The listing builds one solid part. Answer for the finished solid, in the listing's coordinates (mm). Face numbers are marked on the shaded views. A direction names the side the tool comes from. Coordinates: 2 decimals unless noted, no trailing zeros. Order: outer loops, then holes, each group sorted by start corner. A loop starts at its lowest first (then second) coordinate and runs counter-clockwise, first axis right, second up. Notation, with made-up numbers: (71, 17) -> (75, 17) arc R15 ccw to (75, 35) -> close; hole circle Ø4 at (63, 27.5). An arc over 180 degrees is marked (long way). Return JSON: item names as keys, results as strings.
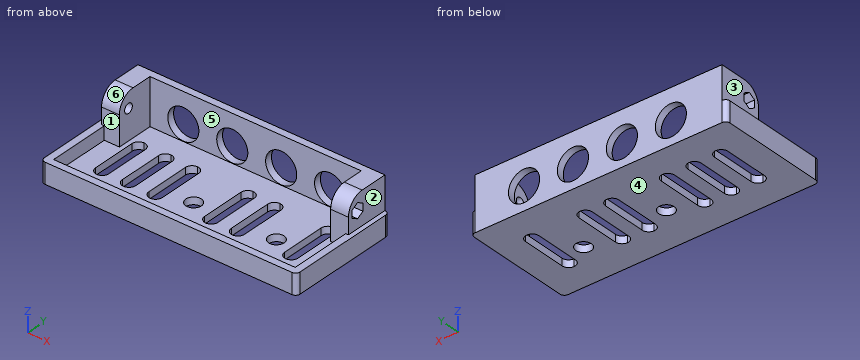
```python
from build123d import *

# Parameters (mm, degrees)
F0_W      = 115
F0_H      = 51
F0_R      = 3.5
F1_DEPTH  = 3.2
F3_DEPTH  = 24
F5_DEPTH  = 6
F6_R      = 2.125
F7_DEPTH  = 113.001
F8_R      = 7.5
F9_R      = 2
F10_R     = 7
F11_DEPTH = 5
F13_DEPTH = 4


# Not quite as in the source:
# - a pattern or mirror of a feature is missing from the dataset's text; its kind, count and spacing are read off the source's solid


with BuildPart() as f1:
    # F0 (on Top) → F1 (new body)
    with BuildSketch(Plane.XY):
        Rectangle(F0_W, F0_H)
        with BuildLine():
            Line((-39.5, 10), (-39.5, -10))
            ThreePointArc((-39.5, -10), (-40.3786796564, -12.1213203436), (-42.5, -13))
            ThreePointArc((-42.5, -13), (-44.6213203436, -12.1213203436), (-45.5, -10))
            Line((-45.5, -10), (-45.5, 10))
            ThreePointArc((-45.5, 10), (-44.6213203436, 12.1213203436), (-42.5, 13))
            ThreePointArc((-42.5, 13), (-40.3786796564, 12.1213203436), (-39.5, 10))
        make_face(mode=Mode.SUBTRACT)
        with Locations((-5.112, -5.5)):
            Circle(F0_R, mode=Mode.SUBTRACT)
        with Locations((32.1, -5.5)):
            Circle(F0_R, mode=Mode.SUBTRACT)
        with BuildLine():
            Line((-27.5, 10), (-27.5, -10))
            ThreePointArc((-27.5, -10), (-28.3786796564, -12.1213203436), (-30.5, -13))
            ThreePointArc((-30.5, -13), (-32.6213203436, -12.1213203436), (-33.5, -10))
            Line((-33.5, -10), (-33.5, 10))
            ThreePointArc((-33.5, 10), (-32.6213203436, 12.1213203436), (-30.5, 13))
            ThreePointArc((-30.5, 13), (-28.3786796564, 12.1213203436), (-27.5, 10))
        make_face(mode=Mode.SUBTRACT)
        with BuildLine():
            Line((-15.5, 10), (-15.5, -10))
            ThreePointArc((-15.5, -10), (-16.3786796564, -12.1213203436), (-18.5, -13))
            ThreePointArc((-18.5, -13), (-20.6213203436, -12.1213203436), (-21.5, -10))
            Line((-21.5, -10), (-21.5, 10))
            ThreePointArc((-21.5, 10), (-20.6213203436, 12.1213203436), (-18.5, 13))
            ThreePointArc((-18.5, 13), (-16.3786796564, 12.1213203436), (-15.5, 10))
        make_face(mode=Mode.SUBTRACT)
        with BuildLine():
            Line((9.5, 10), (9.5, -10))
            ThreePointArc((9.5, -10), (8.6213203436, -12.1213203436), (6.5, -13))
            ThreePointArc((6.5, -13), (4.3786796564, -12.1213203436), (3.5, -10))
            Line((3.5, -10), (3.5, 10))
            ThreePointArc((3.5, 10), (4.3786796564, 12.1213203436), (6.5, 13))
            ThreePointArc((6.5, 13), (8.6213203436, 12.1213203436), (9.5, 10))
        make_face(mode=Mode.SUBTRACT)
        with BuildLine():
            Line((21.5, 10), (21.5, -10))
            ThreePointArc((21.5, -10), (20.6213203436, -12.1213203436), (18.5, -13))
            ThreePointArc((18.5, -13), (16.3786796564, -12.1213203436), (15.5, -10))
            Line((15.5, -10), (15.5, 10))
            ThreePointArc((15.5, 10), (16.3786796564, 12.1213203436), (18.5, 13))
            ThreePointArc((18.5, 13), (20.6213203436, 12.1213203436), (21.5, 10))
        make_face(mode=Mode.SUBTRACT)
        with BuildLine():
            Line((45.5, 10), (45.5, -10))
            ThreePointArc((45.5, -10), (44.6213203436, -12.1213203436), (42.5, -13))
            ThreePointArc((42.5, -13), (40.3786796564, -12.1213203436), (39.5, -10))
            Line((39.5, -10), (39.5, 10))
            ThreePointArc((39.5, 10), (40.3786796564, 12.1213203436), (42.5, 13))
            ThreePointArc((42.5, 13), (44.6213203436, 12.1213203436), (45.5, 10))
        make_face(mode=Mode.SUBTRACT)
    extrude(amount=F1_DEPTH)

    # F2 (on face) → F3 (join)
    with BuildSketch(Plane(origin=(0, 0, 0), x_dir=(1, 0, 0), z_dir=(0, 0, -1))):
        Polygon((-47.5, -5.5), (-55.5, -5.5), (-55.5, -25.5), (55.5, -25.5), (55.5, -5.5), (47.5, -5.5), (47.5, -22.3), (-47.5, -22.3), align=None)
    extrude(amount=-F3_DEPTH)

    # F4 (on face) → F5 (join)
    with BuildSketch(Plane.XY.offset(3.2)):
        Polygon((-55.5, 5.5), (-55.5, 25.5), (-57.5, 25.5), (-57.5, -25.5), (57.5, -25.5), (57.5, 25.5), (55.5, 25.5), (55.5, 5.5), (54.3, 5.5), (54.3, -22.3), (-54.3, -22.3), (-54.3, 5.5), align=None)
    extrude(amount=F5_DEPTH)

    # F6 (on face) → F7 (cut, through all)
    with BuildSketch(Plane.YZ.offset(55.5)):
        with Locations((10.5, 16.7)):
            Circle(F6_R)
    extrude(amount=-F7_DEPTH, mode=Mode.SUBTRACT)

    # F8
    f8_edges = [f1.edges().sort_by_distance(p)[0] for p in [
        (51.5, 5.5, 24),
        (-51.5, 5.5, 24),
    ]]
    fillet(f8_edges, radius=F8_R)

    # F9
    f9_edges = [f1.edges().sort_by_distance(p)[0] for p in [
        (-57.5, -25.5, 4.6),
        (57.5, -25.5, 4.6),
        (57.5, 25.5, 4.6),
        (-57.5, 25.5, 4.6),
    ]]
    fillet(f9_edges, radius=F9_R)

    # F10 (on face) → F11 (cut)
    with BuildSketch(Plane(origin=(0, 25.5, 0), x_dir=(-1, 0, 0), z_dir=(0, 1, 0))):
        with Locations((-33.5, 10.4)):
            Circle(F10_R)
        with Locations((-11.5, 10.4)):
            Circle(F10_R)
        with Locations((10.5, 10.4)):
            Circle(F10_R)
        with Locations((32.5, 10.4)):
            Circle(F10_R)
    extrude(amount=-F11_DEPTH, mode=Mode.SUBTRACT)

    # F12 (on face) → F13 (cut)
    with BuildSketch(Plane(origin=(-55.5, 0, 0), x_dir=(0, -1, 0), z_dir=(-1, 0, 0))):
        Polygon((-7.575, 15.0112504626), (-7.575, 18.3887495374), (-10.5, 20.0774990748), (-13.425, 18.3887495374), (-13.425, 15.0112504626), (-10.5, 13.3225009252), align=None)
    f13 = extrude(amount=-F13_DEPTH, mode=Mode.SUBTRACT)

    # F13_copies: F13 across plane
    add(f13.mirror(Plane(origin=(0, 0, 0), x_dir=(0, 0, 1), z_dir=(1, 0, 0))), mode=Mode.SUBTRACT)


solid = f1.part
```
Item 1: The part is cut by section B-B on y = 0. Count the separate pieces of the cut face and the enclosed holes in it, plus the area to 3 significant figures.
Answer list:
{"separate pieces": "7", "enclosed holes": "0", "area": "291 mm2"}
Item 2: The part is cut by section C-C on x = 33.5. Determine the outline of the cut face in (y, z), plus the area to 3 significant figures.
Answer list:
{"outline": "(-25.5, 0) -> (-8.71, 0) -> (-8.71, 3.2) -> (-22.3, 3.2) -> (-22.3, 9.2) -> (-25.5, 9.2) -> close; (-2.29, 0) -> (25.5, 0) -> (25.5, 3.4) -> (22.3, 3.4) -> (22.3, 3.2) -> (-2.29, 3.2) -> close; (22.3, 17.4) -> (25.5, 17.4) -> (25.5, 24) -> (22.3, 24) -> close", "area": "184 mm2"}
Item 3: Find the intervals of material crossed by probe 1 along Y at (x, z) = (6, 4); probe 2 along X at (y, z) = (8.5, 8.25); probe 3 along X at (y, z) = (18, 14.5), in increasing order.
Answer list:
{"probe 1": "-25.5 to -22.3, 22.3 to 25.5", "probe 2": "-57.5 to -47.5, 47.5 to 57.5", "probe 3": "-55.5 to -47.5, 47.5 to 55.5"}
Item 4: Flat-ended cylindrical pins translate along their axes: pin 1 (6 mm diameter, centred on x = 22.5, y = 13.5, fed in from +Z); pin 2 (8.5 mm diameter, centred on x = -10.5, z = 10.4, fed in from +Y); pin 3 (3 mm diameter, centred on x = 12, z = 21.5, fed in from -Y); pin 4 (6 mm diameter, centred on y = -2.5, z = 14, fed in from +X). Find the tip coordinate at first contact, or state that the pin passes through.
Answer list:
{"pin 1": "z = 3.2", "pin 2": "y = -22.3", "pin 3": "y = 22.3", "pin 4": "through"}
Item 5: The part is cut by section A-A on x = 11.5. Determine the outline of the cut face in (y, z).
Answer list:
{"outline": "(-25.5, 0) -> (25.5, 0) -> (25.5, 3.4) -> (22.3, 3.4) -> (22.3, 3.2) -> (-22.3, 3.2) -> (-22.3, 9.2) -> (-25.5, 9.2) -> close; (22.3, 17.4) -> (25.5, 17.4) -> (25.5, 24) -> (22.3, 24) -> close"}
Item 6: The part is cut by section D-D on y = -20. Determine the outline of the cut face in (x, z).
Answer list:
{"outline": "(-57.5, 0) -> (57.5, 0) -> (57.5, 9.2) -> (54.3, 9.2) -> (54.3, 3.2) -> (-54.3, 3.2) -> (-54.3, 9.2) -> (-57.5, 9.2) -> close"}
Item 7: Which of the six approach directions +Z, -Z, +X, -X, +Y, -Y give full straight-line access (tool end or side, diameter ignored) to the marked faces 1, 2 and 3?
Answer list:
{"face 1": "+Z", "face 2": "+Z, +X, +Y, -Y", "face 3": "+Z, -X, +Y, -Y"}
Item 8: Determine the mould class of the marked faces 4, 5 and 6 for opening direction Y: pulls with the +Y half, pulls with the -Y half, needs draft (parallel to the pull), parting line crosses it, or undercut.
Answer list:
{"face 4": "needs draft", "face 5": "undercut", "face 6": "pulls with the -Y half"}
